from build123d import *

# Parameters (mm, degrees)
EXTRUDE_1_DEPTH = 10


with BuildPart() as part:
    # 草图1 → 凸台-拉伸1 (new body)
    with BuildSketch(Plane(origin=(0, 0, 0), x_dir=(0, 0, -1), z_dir=(1, 0, 0))):
        with BuildLine():
            Line((7.589042449, 29.024238745), (-130, 65))
            Line((-130, 65), (-530, 65))
            Line((-530, 65), (-530, -65))
            Line((-530, -65), (-130, -65))
            Line((-130, -65), (7.589042449, -29.024238745))
            ThreePointArc((7.589042449, -29.024238745), (30, 0), (7.589042449, 29.024238745))
        make_face()
    extrude(amount=EXTRUDE_1_DEPTH)


solid = part.part
The model under review builds one solid part; all positions refer to its coordinate system, in mm. Give positions to 0.01 mm unless a question says otherwise; leave off trailing zeros. Write each loop counter-clockwise with the first axis right and the second up, starting at its lowest first coordinate (ties: lowest second). Pieces come first, ordered by that corner, then holes.
1. Add section B-B, the plane y = -54. Write out the cut boundary in (x, z), plus the area to 3 significant figures.
2. Add section A-A, the plane x = 5.25. Write out the cut boundary in (y, z), plus the area to 3 significant figures.
3. Add section C-C, the plane z = 87.5. Write out the cut boundary in (x, y).
4. Wall thickness on L1, parallel to Y at x = 4.5, z = 122; L2, parallel to Z at x = 5.5, y = -18; L3, parallel to Y at x = 9.5, z = 13.5: over which ranges is each line inside the solid? List them lowest first.
Worked answers:
1. outline: (0, 87.93) - (10, 87.93) - (10, 530) - (0, 530) - close
1. area: 4,420 mm2
2. outline: (-65, 130) - (-29.02, -7.59) arc R30 ccw to (29.02, -7.59) - (65, 130) - (65, 530) - (-65, 530) - close
2. area: 65,900 mm2
3. outline: (0, -53.89) - (10, -53.89) - (10, 53.89) - (0, 53.89) - close
4. L1: y = -62.91 to 62.91
4. L2: z = -24 to 530
4. L3: y = -34.54 to 34.54
